Input: part model. Units: mm. Frame: model coordinates. Face numbers are marked on the shaded views. A direction names the side the tool comes from. Round coordinates to 2 decimals unless told otherwise and drop trailing zeros. Order: outer loops, then holes, each group sorted by start corner. A loop starts at its lowest first (then second) coordinate and runs counter-clockwise, first axis right, second up. Notation, with made-up numbers: (51.5, -5.75) -> (104.5, -5.75) arc R29 ccw to (104.5, 21.25) -> close; hole circle Ø9 at (-17, 17.5). An arc over 180 degrees is marked (long way). Use a Markdown table: item, result.
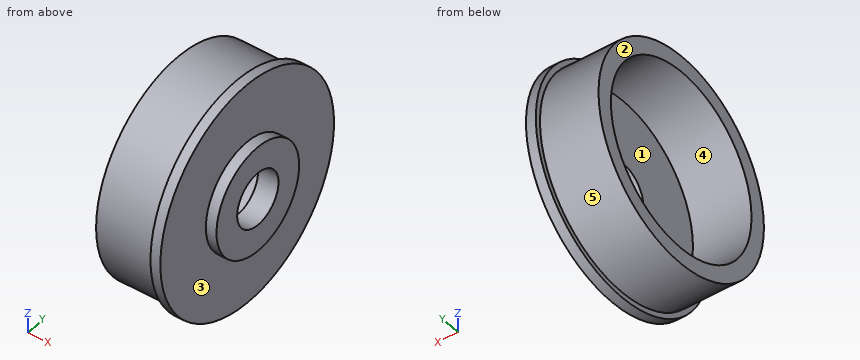
from build123d import *

# Parameters (mm, degrees)
F0_W   = 11
F0_H   = 3
F0_W_2 = 2
F0_H_2 = 5


with BuildPart() as f1:
    # F0 (on Front) → F1 (revolve)
    with BuildSketch(Plane.XZ):
        with Locations((-5.5, 18.5)):
            Rectangle(F0_W, F0_H)
        Polygon((0, 17), (0, 5), (1.85, 5), (1.85, 10), (1.85, 21), (0, 21), (0, 20), align=None)
        with Locations((2.85, 7.5)):
            Rectangle(F0_W_2, F0_H_2)
    revolve(axis=Axis((4.390737, 0, 0), (1, 0, 0)))


solid = f1.part
1) Pin query (flat end, axial travel): pin 1 Ø11.5 at (y, z) = (0, 0) entering from -X; pin 2 Ø5 at (x, z) = (-1, -10.5) entering from -Y; pin 3 Ø1 at (x, z) = (-4.5, -7) entering from -Y. Return the tip coordinate at first contact, or that it passes through.
Results found:
| item | result |
|---|---|
| pin 1 | stops at x = 0 |
| pin 2 | stops at y = -19.33 |
| pin 3 | stops at y = -18.91 |
2) Pull-direction query (Z, two-part tool) for the marked faces 3, 4 and 5; classes: +Z half, -Z half, draft (parallel to the pull), parting line (faces both ways), or undercut.
Results found:
| item | result |
|---|---|
| face 3 | draft |
| face 4 | undercut |
| face 5 | parting line |
3) Cut plane C-C on x = -9.25. Return loops of the section in (y, z).
Results found:
| item | result |
|---|---|
| outline | circle Ø40 at (0, 0); hole circle Ø34 at (0, 0) |
4) Cut plane D-D on z = 13.5. Return loops of the section in (x, y), and give its area (3 significant figures).
Results found:
| item | result |
|---|---|
| outline | (-11, -14.76) -> (0, -14.76) -> (0, -16.09) -> (1.85, -16.09) -> (1.85, 16.09) -> (0, 16.09) -> (0, 14.76) -> (-11, 14.76) -> (-11, 10.33) -> (0, 10.33) -> (0, -10.33) -> (-11, -10.33) -> close |
| area | 157 mm² |
5) Cut plane A-A on y = 0. Return loops of the section in (x, z), and give its area (3 significant figures).
Results found:
| item | result |
|---|---|
| outline | (-11, -20) -> (0, -20) -> (0, -21) -> (1.85, -21) -> (1.85, -10) -> (3.85, -10) -> (3.85, -5) -> (0, -5) -> (0, -17) -> (-11, -17) -> close; (-11, 17) -> (0, 17) -> (0, 5) -> (3.85, 5) -> (3.85, 10) -> (1.85, 10) -> (1.85, 21) -> (0, 21) -> (0, 20) -> (-11, 20) -> close |
| area | 145 mm² |
6) Line query: L1, parallel to Z at x = 1.45, y = 0; L2, parallel to Z at x = 2.35, y = 0; L3, parallel to Y at x = -6.25, z = 0. Output: solid intervals per line, ascending. Write a range as [from, to].
Results found:
| item | result |
|---|---|
| L1 | z = [-21, -5], [5, 21] |
| L2 | z = [-10, -5], [5, 10] |
| L3 | y = [-20, -17], [17, 20] |
7) Set-up query: the marked faces 1 and 2. Return all of +Z, -Z, +X, -X, +Y, -Y with unobstructed straight access to the full face (end or side cutting, diameter ignored); none if empty.
Results found:
| item | result |
|---|---|
| face 1 | -X |
| face 2 | +Z, -Z, -X, +Y, -Y |
